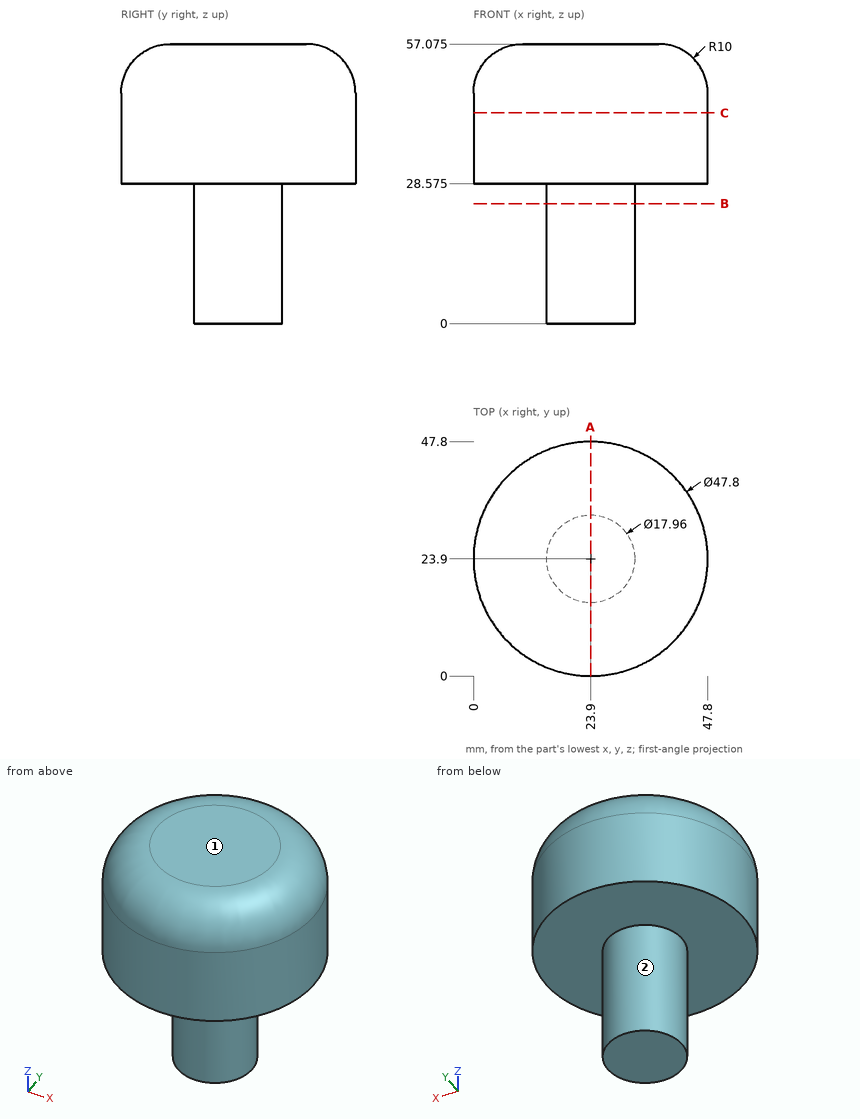
Design review of the part shown in the three views and the two pictorial views. Dimensions are in mm from the part's minimum x, y and z. A direction names the side the tool comes from. Round coordinates to 2 decimals unless told otherwise and drop trailing zeros. Write each loop counter-clockwise with the first axis right and the second up, starting at its lowest first coordinate (ties: lowest second). Pieces come first, ordered by that corner, then holes. Notation, with made-up numbers: (46.25, 3) -> (78.25, 3) arc R11 cw to (78.25, 14) -> close; hole circle Ø7 at (-40, -17.5). An arc over 180 degrees is marked (long way). Use one line per item in the form item = value.
1) Tool access review of the marked faces 1 and 2: name each direction out of +Z, -Z, +X, -X, +Y, -Y from which nothing blocks a thin tool from reaching the whole face with its end or side.
Found:
face_1 = +Z, +X, -X, +Y, -Y
face_2 = -Z
2) Take a section at C-C, the plane z = 43. Write out the cut boundary in (x, y).
Found:
outline = circle Ø47.8 at (23.9, 23.9)
3) Take a section at B-B, the plane z = 24.5. Write out the cut boundary in (x, y).
Found:
outline = circle Ø17.96 at (23.9, 23.9)
4) To check wall thickness, follow L1, parallel to Z at x = 22.5, y = 34.5 (3 decimals); L2, parallel to X at y = 31, z = 23; L3, parallel to Y at x = 36.5, z = 44. State the ranges of each line that lie inside material, in increasing order. Write a range as from..to.
Found:
L1 = 28.575..57.075
L2 = 18.4..29.4
L3 = 3.59..44.21
5) Clearance check with flat-ended pins moving along their axes: pin 1 (12 mm diameter, centred on x = 36, z = 50.5, fed in from +Y); pin 2 (5 mm diameter, centred on y = 32.5, z = 10, fed in from +X); pin 3 (1 mm diameter, centred on y = 29.5, z = 6, fed in from -X). State where each tip first meets the part, or that it passes through.
Found:
pin_1 = 46.82
pin_2 = 30.49
pin_3 = 16.51
6) Take a section at A-A, the plane x = 23.9. Write out the cut boundary in (y, z) (3 decimals).
Found:
outline = (0, 28.575) -> (14.92, 28.575) -> (14.92, 0) -> (32.88, 0) -> (32.88, 28.575) -> (47.8, 28.575) -> (47.8, 47.075) arc R10 ccw to (37.8, 57.075) -> (10, 57.075) arc R10 ccw to (0, 47.075) -> close
